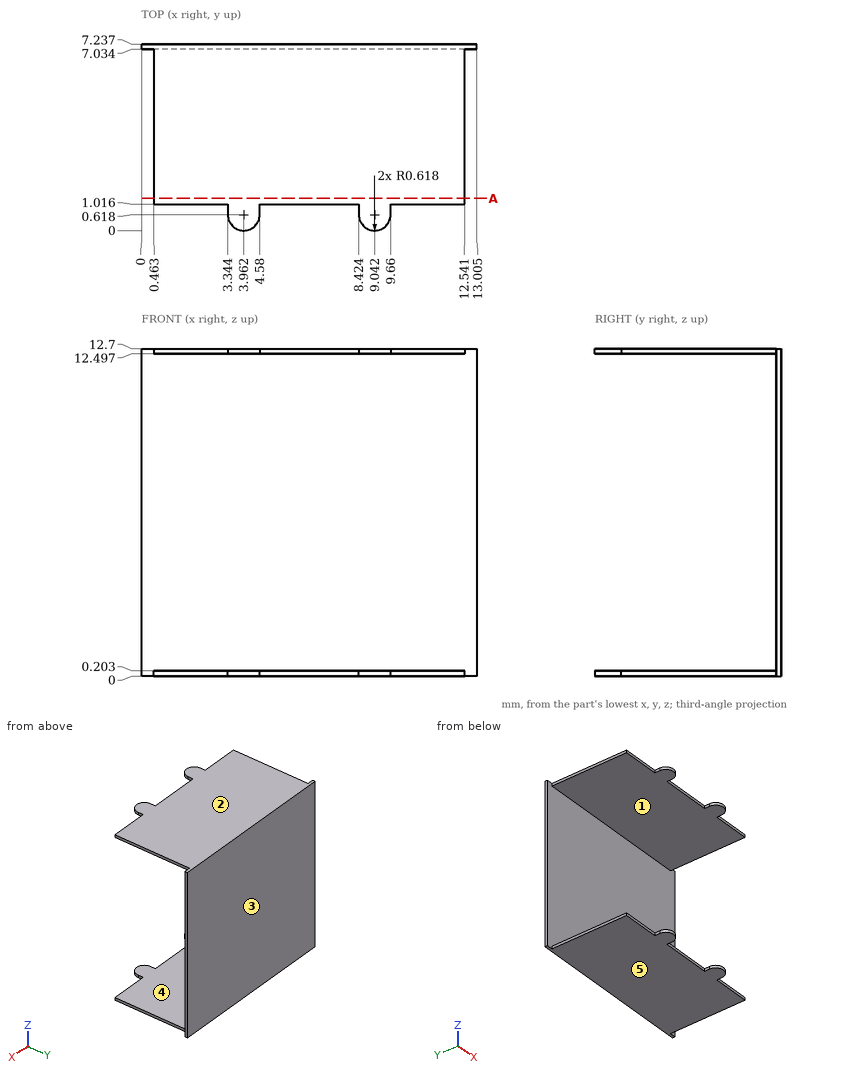
Geometry check sheet. Reference: drawing and pictorial views, mm from the part's lowest x, y, z. A direction names the side the tool comes from. Give positions to 0.01 mm unless a question says otherwise; leave off trailing zeros. Loops run counter-clockwise (first coordinate to the right, second up) from the corner with the lowest first, then second, coordinate; pieces in that order, holes last. Notation, with made-up numbers: M 64,41 L 87,41 A18 cw 87,71 Z; hole C 0.25,-26.5 d3. An arc over 180 degrees is marked long. Use a Markdown table: item, result. Add a question column.
Q1. Scan lines: line 1 along Z through (x, y) = (11, 3); line 2 along Y through (x, z) = (2.5, 1) (1 decimal). Record each from-to range of solid material in increasing order. Write a range as [from, to].
Q2. Sectioned sample at A-A, the plane y = 1.25. Record the cut outline in (x, z).
Q3. Tool access check on the marked faces 1 and 2. Record the directions out of +Z, -Z, +X, -X, +Y, -Y that give a thin tool (end or side, any length) a straight path to the whole face; none if there is none.
Q4. Go/stop test with flat-tipped pins: pin 1 (5 mm diameter, centred on x = 4, z = 2.5, fed in from -Y); pin 2 (1.5 mm diameter, centred on x = 4, z = 10, fed in from -Y); pin 3 (5 mm diameter, centred on x = 1.5, z = 2, fed in from -Y). Record where each tip stops, or that it passes through.
Q5. Mould release check, pull along Z, two halves, no side actions. Record for the marked faces 3, 4 and 5: pulls with the +Z half, pulls with the -Z half, needs draft (parallel to the pull), parting line crosses it, or undercut.
Verdict:
| question | item | result |
|---|---|---|
| 1 | line 1 | [0, 0.2], [12.5, 12.7] |
| 1 | line 2 | [7, 7.2] |
| 2 | outline | M 0.46,0 L 12.54,0 L 12.54,0.2 L 0.46,0.2 Z; M 0.46,12.5 L 12.54,12.5 L 12.54,12.7 L 0.46,12.7 Z |
| 3 | face 1 | +X, -X, -Y |
| 3 | face 2 | +Z, +X, -X, +Y, -Y |
| 4 | pin 1 | y = 0 |
| 4 | pin 2 | y = 7.03 |
| 4 | pin 3 | y = 1.02 |
| 5 | face 3 | needs draft |
| 5 | face 4 | undercut |
| 5 | face 5 | pulls with the -Z half |
